Print and shaded views of the part. All mm, measured from the part's lowest x, y and z. A direction names the side the tool comes from. Round coordinates to 2 decimals unless told otherwise and drop trailing zeros. Loops run counter-clockwise (first coordinate to the right, second up) from the corner with the lowest first, then second, coordinate; pieces in that order, holes last. Notation, with made-up numbers: (-28.75, -27.75) -> (16.25, -27.75) arc R13 ccw to (16.25, -5.75) -> close; hole circle Ø8 at (86.25, 12). An arc over 180 degrees is marked (long way). Use a Markdown table: item, result.
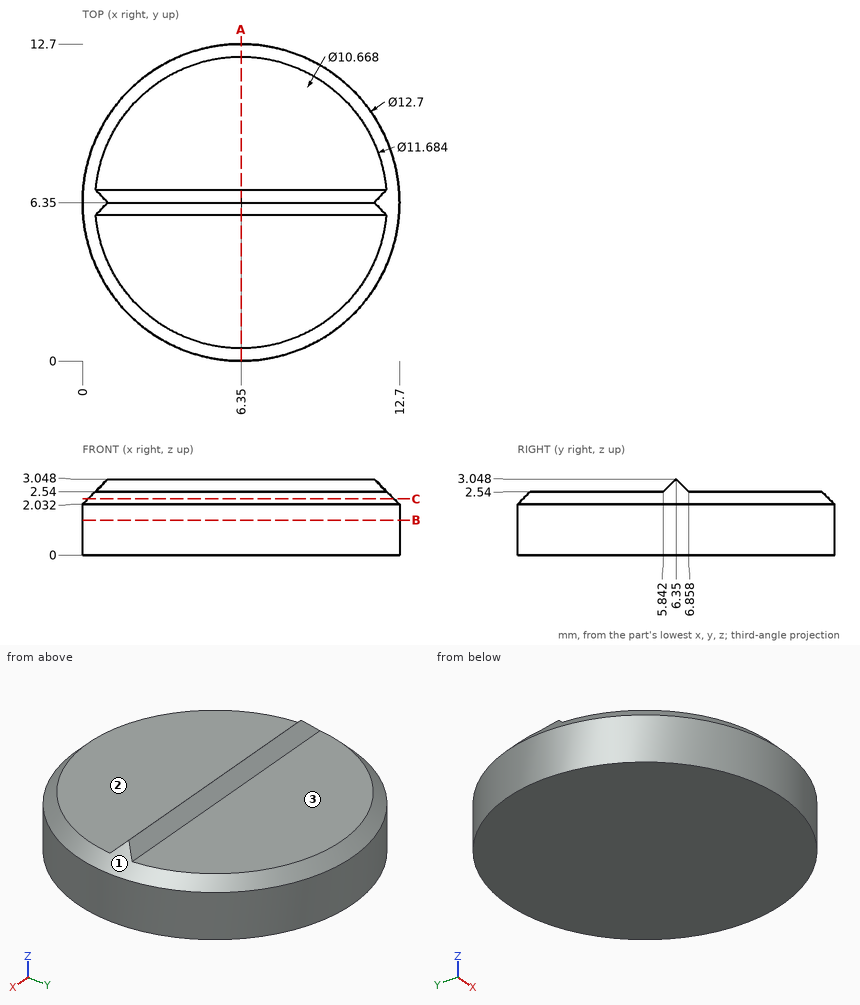
Q1. Drill centre lines: L1, parallel to Z at x = 3.5, y = 11; L2, parallel to X at y = 4, z = 1.1; L3, parallel to X at y = 9, z = 1.25. Where is each one in solid material? Low to high. Write a range as from..to.
Results list:
| item | result |
|---|---|
| L1 | z = 0..2.54 |
| L2 | x = 0.45..12.25 |
| L3 | x = 0.58..12.12 |
Q2. Band-saw the part on A-A, the plane x = 6.35. Give the cut face in (y, z), plus the area to 3 significant figures.
Results list:
| item | result |
|---|---|
| outline | (0, 0) -> (12.7, 0) -> (12.7, 2.03) -> (12.19, 2.54) -> (6.86, 2.54) -> (6.35, 3.05) -> (5.84, 2.54) -> (0.51, 2.54) -> (0, 2.03) -> close |
| area | 32.3 mm² |
Q3. Tool access for the marked faces 1, 2 and 3: list every direction of +Z, -Z, +X, -X, +Y, -Y with a clear straight run to the whole face (end or side of a thin tool).
Results list:
| item | result |
|---|---|
| face 1 | +Z |
| face 2 | +Z, +X, -X, -Y |
| face 3 | +Z, +X, -X, +Y |
Q4. Band-saw the part on C-C, the plane z = 2.25. Give the cut face in (x, y), plus the area to 3 significant figures.
Results list:
| item | result |
|---|---|
| outline | circle Ø12.26 at (6.35, 6.35) |
| area | 118 mm² |
Q5. Band-saw the part on B-B, the plane z = 1.4. Give the cut face in (x, y), plus the area to 3 significant figures.
Results list:
| item | result |
|---|---|
| outline | circle Ø12.7 at (6.35, 6.35) |
| area | 127 mm² |
Q6. Flat gauge pins, fed straight in: pin 1 (4.5 mm diameter, centred on x = 7, y = 8.5, fed in from +Z); pin 2 (1.6 mm diameter, centred on x = 9, y = 4, fed in from +Z); pin 3 (1.5 mm diameter, centred on x = 7.5, z = 2.5, fed in from +Y). Where does each tip first touch, or does it go through?
Results list:
| item | result |
|---|---|
| pin 1 | stops at z = 3.05 |
| pin 2 | stops at z = 2.54 |
| pin 3 | stops at y = 12.67 |
